```python
from build123d import *

# Parameters (mm, degrees)
SKETCH1_R           = 1.5875
BOSS_EXTRUDE1_DEPTH = 6.35
FILLET1_R           = 3.175
SKETCH2_R           = 1.5875
TIES_HOLE_DEPTH     = 34.893775609


with BuildPart() as part:
    # Sketch1 → Boss-Extrude1 (new body)
    with BuildSketch(Plane(origin=(0, 0, 0), x_dir=(1, 0, 0), z_dir=(0, 1, 0))):
        with BuildLine():
            Line((-27.305, 5.715), (-20.955, 5.715))
            Line((-20.955, 5.715), (-20.955, 10.4775))
            ThreePointArc((-20.955, 10.4775), (-19.3675, 12.065), (-20.955, 13.6525))
            Line((-20.955, 13.6525), (-20.955, 20.0025))
            ThreePointArc((-20.955, 20.0025), (-19.3675, 21.59), (-20.955, 23.1775))
            Line((-20.955, 23.1775), (-20.955, 24.765))
            Line((-20.955, 24.765), (-11.43, 24.765))
            Line((-11.43, 24.765), (-11.43, 23.1775))
            ThreePointArc((-11.43, 23.1775), (-13.0175, 21.59), (-11.43, 20.0025))
            Line((-11.43, 20.0025), (-11.43, 13.6525))
            ThreePointArc((-11.43, 13.6525), (-13.0175, 12.065), (-11.43, 10.4775))
            Line((-11.43, 10.4775), (-11.43, 5.715))
            Line((-11.43, 5.715), (27.305, 5.715))
            Line((27.305, 5.715), (27.305, -5.715))
            Line((27.305, -5.715), (-27.305, -5.715))
            Line((-27.305, -5.715), (-27.305, 5.715))
        make_face()
        with Locations(Location((-24.13, 0, 0), (0, 0, 270))):
            Circle(SKETCH1_R, mode=Mode.SUBTRACT)
        with Locations(Location((24.13, 0, 0), (0, 0, 270))):
            Circle(SKETCH1_R, mode=Mode.SUBTRACT)
    extrude(amount=BOSS_EXTRUDE1_DEPTH)

    # Fillet1
    fillet1_edges = [part.edges().sort_by_distance(p)[0] for p in [
        (-20.955, 3.175, -5.715),
        (-11.43, 3.175, -5.715),
    ]]
    fillet(fillet1_edges, radius=FILLET1_R)

    # Sketch2 → ties hole (cut, through all)
    with BuildSketch(Plane(origin=(0, 0, -5.715), x_dir=(-1, 0, 0), z_dir=(0, 0, -1))):
        with Locations((4.445, 3.175)):
            Circle(SKETCH2_R)
    extrude(amount=-TIES_HOLE_DEPTH, mode=Mode.SUBTRACT)


solid = part.part
```
Part model, mm, in its own coordinate system. A direction names the side the tool comes from. Give positions to 0.01 mm unless a question says otherwise; leave off trailing zeros. Loops run counter-clockwise (first coordinate to the right, second up) from the corner with the lowest first, then second, coordinate; pieces in that order, holes last. Notation, with made-up numbers: M 12.5,15.25 L 17.5,15.25 A30 ccw 17.5,48.25 Z; hole C 18.25,3 d2. An arc over 180 degrees is marked long. Return JSON: item names as keys, results as strings.
1) 3-axis set-ups, long thin cutter, end or side, ignore diameter. For faces 4 (the face through (9, 3, -5.715)), 5 (the face through (-13.017, 3.131, -21.625)), 6 (the face through (-26, 3, -5.715)): which of +Z, -Z, +X, -X, +Y, -Y reach the whole face in a straight line?
Calculated:
{"face 4": "-Z, +X, +Y, -Y", "face 5": "+X, +Y, -Y", "face 6": "-Z, -X, +Y, -Y"}
2) Saw through at D-D, the plane z = -21.59. List the corners of the cut face in (x, y), then the cut area to 3 significant figures.
Calculated:
{"outline": "M -19.37,0 L -13.02,0 L -13.02,6.35 L -19.37,6.35 Z", "area": "40.3 mm2"}
3) Saw through at A-A, the plane y = 5.5. Count the separate pieces of the cut face and the enclosed holes in it, then the cut area to 3 significant figures.
Calculated:
{"separate pieces": "1", "enclosed holes": "2", "area": "778 mm2"}
4) Pull direction X, two halves, no side cores. Call faces 1 (the face through (-22.79, 3.13, 0.85)), 2 (the face through (-11.43, 3, -24)), 3 (the face through (-27.305, 3, 0)): released by +X, released by -X, zero draft, split by the parting line, or undercut.
Calculated:
{"face 1": "undercut", "face 2": "released by +X", "face 3": "released by -X"}
5) Flat gauge pins, fed straight in: pin 1 Ø3 at (y, z) = (4.5, -15.5) entering from +X; pin 2 Ø2.5 at (x, y) = (-25.5, 2.5) entering from -Z (3 decimals); pin 3 Ø0.8 at (y, z) = (4.5, -24) entering from -X (3 decimals); pin 4 Ø3 at (x, y) = (-4.445, 3.175) entering from -Z. Where does each tip first touch, or does it go through?
Calculated:
{"pin 1": "stops at x = -11.43", "pin 2": "stops at z = -5.715", "pin 3": "stops at x = -20.955", "pin 4": "passes through"}
6) Drill centre lines: line 1 (X direction, y = 3, z = 0) (1 decimal); line 2 (Z direction, x = -12.5, y = 5.5) (3 decimals); line 3 (X direction, y = 2.25, z = 0) (1 decimal). Where is each one in solid material? Low to high.
Calculated:
{"line 1": "x = -27.3 to -25.7, -22.5 to -6, -2.9 to 22.5, 25.7 to 27.3", "line 2": "z = -24.765 to -22.763, -20.417 to -13.238, -10.892 to 5.715", "line 3": "x = -27.3 to -25.7, -22.5 to -5.7, -3.2 to 22.5, 25.7 to 27.3"}
